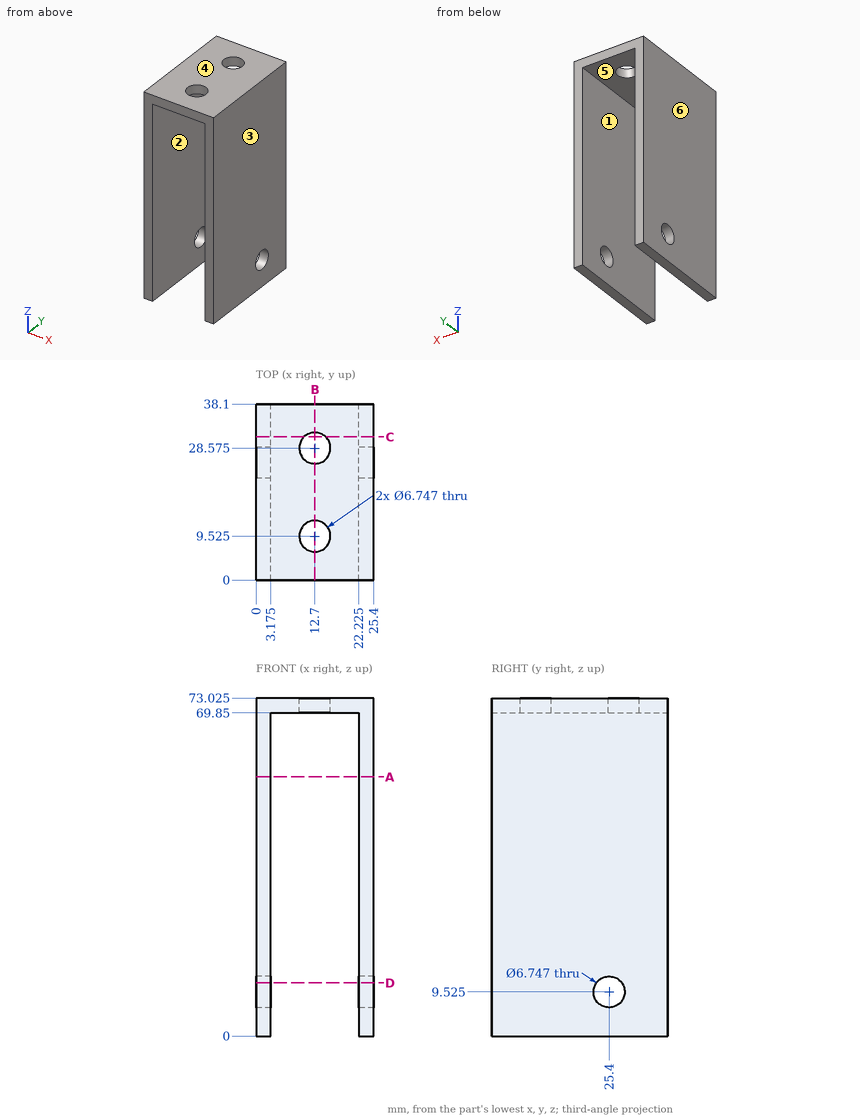
Geometry check sheet. Reference: drawing and pictorial views, mm from the part's lowest x, y, z. A direction names the side the tool comes from. Round coordinates to 2 decimals unless told otherwise and drop trailing zeros. Loops run counter-clockwise (first coordinate to the right, second up) from the corner with the lowest first, then second, coordinate; pieces in that order, holes last. Notation, with made-up numbers: (54.5, 61.5) - (58.5, 61.5) arc R26 ccw to (58.5, 78.5) - close; hole circle Ø6 at (-14.75, 51). An arc over 180 degrees is marked (long way). Use a Markdown table: item, result. Add a question column.
1. Section check C-C, the plane y = 31. Record the boundary of the cut face in (x, z) (3 decimals).
2. Gauge pin test, flat ends, axial feed: pin 1 (9.5 mm diameter, centred on x = 9.5, y = 21.5, fed in from -Z); pin 2 (4 mm diameter, centred on y = 25.4, z = 9.525, fed in from -X) (1 decimal). Record the tip position at first contact, or that the pin passes through.
3. Release check for a two-part mould opening along X. For the marked faces 1, 2, 3 and 4 record: released by +X, released by -X, zero draft, split by the parting line, or undercut.
4. Thickness scan on probe 1 along Y at (x, z) = (12.7, 72.15); probe 2 along X at (y, z) = (16.5, 34.5) (3 decimals); probe 3 along Z at (x, y) = (16.25, 8) (3 decimals). Record the ranges inside material, lowest first. Write a range as [from, to].
5. Access from +Z, -Z, +X, -X, +Y, -Y to the whole of each face (thin tool, end or side, straight path). Record for the marked faces 5 and 6.
6. Section check D-D, the plane z = 11.5. Record the boundary of the cut face in (x, y) (3 decimals).
7. Section check A-A, the plane z = 56. Record the boundary of the cut face in (x, y) (3 decimals).
8. Section check B-B, the plane x = 12.7. Give the number of separate pieces and of enclosed holes in the cut face, plus the area to 3 significant figures.
Checks:
| question | item | result |
|---|---|---|
| 1 | outline | (0, 0) - (3.175, 0) - (3.175, 69.85) - (10.355, 69.85) - (10.355, 73.025) - (0, 73.025) - close; (15.045, 69.85) - (22.225, 69.85) - (22.225, 0) - (25.4, 0) - (25.4, 73.025) - (15.045, 73.025) - close |
| 2 | pin 1 | stops at z = 69.85 |
| 2 | pin 2 | passes through |
| 3 | face 1 | undercut |
| 3 | face 2 | undercut |
| 3 | face 3 | released by +X |
| 3 | face 4 | zero draft |
| 4 | probe 1 | y = [0, 6.15], [12.9, 25.2], [31.95, 38.1] |
| 4 | probe 2 | x = [0, 3.175], [22.225, 25.4] |
| 4 | probe 3 | z = [69.85, 73.025] |
| 5 | face 5 | -Z, +Y, -Y |
| 5 | face 6 | +Z, -Z, -X, +Y, -Y |
| 6 | outline | (0, 0) - (3.175, 0) - (3.175, 22.665) - (0, 22.665) - close; (0, 28.135) - (3.175, 28.135) - (3.175, 38.1) - (0, 38.1) - close; (22.225, 0) - (25.4, 0) - (25.4, 22.665) - (22.225, 22.665) - close; (22.225, 28.135) - (25.4, 28.135) - (25.4, 38.1) - (22.225, 38.1) - close |
| 7 | outline | (0, 0) - (3.175, 0) - (3.175, 38.1) - (0, 38.1) - close; (22.225, 0) - (25.4, 0) - (25.4, 38.1) - (22.225, 38.1) - close |
| 8 | separate pieces | 3 |
| 8 | enclosed holes | 0 |
| 8 | area | 78.1 mm^2 |
